```python
from build123d import *

# Parameters (mm, degrees)
SKETCH1_R           = 12.5
BOSS_EXTRUDE1_DEPTH = 8
SKETCH2_R           = 6.5
CUT_EXTRUDE1_DEPTH  = 4
SKETCH4_R           = 2
CUT_EXTRUDE3_DEPTH  = 4
SKETCH5_W           = 4
SKETCH5_H           = 6
CUT_EXTRUDE4_DEPTH  = 3
SKETCH3_R           = 1
CUT_EXTRUDE2_DEPTH  = 20.403607912
CHAMFER1_SIZE       = 1
CHAMFER2_SIZE       = 1


with BuildPart() as part:
    # Sketch1 → Boss-Extrude1 (new body)
    with BuildSketch(Plane(origin=(0, 0, 0), x_dir=(1, 0, 0), z_dir=(0, 1, 0))):
        with Locations(Location((0, 0, 0), (0, 0, 270))):
            Circle(SKETCH1_R)
    extrude(amount=BOSS_EXTRUDE1_DEPTH)

    # Sketch2 → Cut-Extrude1 (cut)
    with BuildSketch(Plane(origin=(0, 8, 0), x_dir=(1, 0, 0), z_dir=(0, 1, 0))):
        with Locations(Location((0, 0, 0), (0, 0, 270))):
            Circle(SKETCH2_R)
    extrude(amount=-CUT_EXTRUDE1_DEPTH, mode=Mode.SUBTRACT)

    # Sketch4 → Cut-Extrude3 (cut)
    with BuildSketch(Plane(origin=(0, 0, 0), x_dir=(-1, 0, 0), z_dir=(0, -1, 0))):
        with Locations(Location((0, 0, 0), (0, 0, 90))):
            Circle(SKETCH4_R)
    extrude(amount=-CUT_EXTRUDE3_DEPTH, mode=Mode.SUBTRACT)

    # Sketch5 → Cut-Extrude4 (cut)
    with BuildSketch(Plane(origin=(0, 0, 0), x_dir=(-1, 0, 0), z_dir=(0, -1, 0))):
        with Locations((0, -6.25)):
            Rectangle(SKETCH5_W, SKETCH5_H)
        Polygon((-10, -3.25), (-2, -3.25), (-2, 4e-09), (-2, 3.25), (-10, 3.25), align=None)
        with BuildLine():
            Line((-2, -3.25), (2, -3.25))
            Line((2, -3.25), (2, 0))
            ThreePointArc((2, 0), (-2e-09, -2), (-2, 4e-09))
            Line((-2, 4e-09), (-2, -3.25))
        make_face()
        with Locations((0, 6.25)):
            Rectangle(SKETCH5_W, SKETCH5_H)
        Polygon((2, -3.25), (10, -3.25), (10, 3.25), (2, 3.25), (2, 0), align=None)
        with BuildLine():
            ThreePointArc((-2, 4e-09), (2e-09, 2), (2, 0))
            Line((2, 0), (2, 3.25))
            Line((2, 3.25), (-2, 3.25))
            Line((-2, 3.25), (-2, 4e-09))
        make_face()
    extrude(amount=-CUT_EXTRUDE4_DEPTH, mode=Mode.SUBTRACT)

    # Sketch3 → Cut-Extrude2 (cut, through all)
    with BuildSketch(Plane(origin=(0, 8, 0), x_dir=(1, 0, 0), z_dir=(0, 1, 0))):
        with Locations(Location((7.778174593, 7.778174593, 0), (0, 0, 270))):
            Circle(SKETCH3_R)
        with Locations(Location((7.778174593, -7.778174593, 0), (0, 0, 270))):
            Circle(SKETCH3_R)
        with Locations(Location((-7.778174593, -7.778174593, 0), (0, 0, 270))):
            Circle(SKETCH3_R)
        with Locations(Location((-7.778174593, 7.778174593, 0), (0, 0, 270))):
            Circle(SKETCH3_R)
    extrude(amount=-CUT_EXTRUDE2_DEPTH, mode=Mode.SUBTRACT)

    # Chamfer1
    # the kernel refuses this chamfer: 1 mm, written as the material it takes off along each edge
    with BuildSketch(Plane(origin=(0, 0, 0), x_dir=(0, 0, 1), z_dir=(-1, 0, 0))) as chamfer1_piece_1:
        Polygon((12.5, CHAMFER1_SIZE), (12.5 - CHAMFER1_SIZE, 0), (12.5, 0), align=None)
    revolve(axis=Axis((0, 0, 0), (0, 1, 0)), mode=Mode.SUBTRACT)
    with BuildSketch(Plane(origin=(0, 8, 0), x_dir=(0, 0, 1), z_dir=(-1, 0, 0))) as chamfer1_piece_2:
        Polygon((12.5, -CHAMFER1_SIZE), (12.5 - CHAMFER1_SIZE, 0), (12.5, 0), align=None)
    revolve(axis=Axis((0, 8, 0), (0, 1, 0)), mode=Mode.SUBTRACT)
    with BuildSketch(Plane(origin=(0, 8, 0), x_dir=(0, 0, 1), z_dir=(-1, 0, 0))) as chamfer1_piece_3:
        Polygon((6.5 + CHAMFER1_SIZE, 0), (6.5, -CHAMFER1_SIZE), (6.5, 0), align=None)
    revolve(axis=Axis((0, 8, 0), (0, 1, 0)), mode=Mode.SUBTRACT)

    # Chamfer2
    chamfer2_edges = [part.edges().sort_by_distance(p)[0] for p in [
        (2, 1.5, -3.25),
        (-2, 1.5, -3.25),
        (-2, 1.5, 3.25),
        (2, 1.5, 3.25),
    ]]
    chamfer(chamfer2_edges, length=CHAMFER2_SIZE)


solid = part.part
```
Read the model definition and answer for the solid it produces. Units are mm, in the model's axes. A direction names the side the tool comes from. Give positions to 0.01 mm unless a question says otherwise; leave off trailing zeros. Write each loop counter-clockwise with the first axis right and the second up, starting at its lowest first coordinate (ties: lowest second). Pieces come first, ordered by that corner, then holes. Notation, with made-up numbers: (23, -16.5) - (57, -16.5) arc R18 ccw to (57, -3.5) - close; hole circle Ø7 at (34, 69.25). An arc over 180 degrees is marked (long way). Write item = value, one per line. Start each with the question number.
Item 1: A tool of negligible diameter and unlimited length cuts with its end or side. For faces 1 (the cylindrical face through (6.9, 4.1, -7.3)), 2 (the flat face through (0, 1, -9.25)), 3 (the cylindrical face through (-3.955, 5.521, -5.158)), from which of +Z, -Z, +X, -X, +Y, -Y can it reach the whole face along a straight path? Write none if from no direction.
Item 2: Find the intervals of material crossed by probe 1 along X at (y, z) = (4.95, 0); probe 2 along X at (y, z) = (1.75, -7.5); probe 3 along X at (y, z) = (0.75, -7.75), in increasing order. Write a range as [from, to].
Item 3: Find section B-B (z = 0). Give the vertices of the cut face in (x, y).
Item 4: Find section C-C (y = 2.25). Give the vertices of the cut face in (x, z), then the cut area to 3 significant figures.
Item 5: Find section A-A (x = 0). Give the vertices of the cut face in (y, z), then the cut area to 3 significant figures.
Item 6: The mould has two halves that part along X. Classify faces 4 (the flat face through (-8, 8, 0)), 5 (the conical face through (-10.344, 0.16, 5.38)), 6 (the flat face through (2, 1, -7)): +X half, -X half, draft (parallel to the pull), parting line (faces both ways), or undercut.
Item 7: Each of these flat-tipped pins is pushed along its axis until it touches: P1, Ø1.5, axis at y = 1.5, z = 5.5, coming from the +X side; P2, Ø10.5, axis at x = -3, z = 1, coming from the +Y side; P3, Ø6.5, axis at x = 0, z = 0, coming from the -Y side; P4, Ø4, axis at x = -5, y = 1.5, coming from the -Z side. Where does it stop, or does it pass through?
Response:
q1.face_1 = +Y, -Y
q1.face_2 = -Y
q1.face_3 = +Y
q2.probe_1 = [-12.5, -6.5], [6.5, 12.5]
q2.probe_2 = [-10, -8.74], [-6.82, -2], [2, 6.82], [8.74, 10]
q2.probe_3 = [-9.49, -8.78], [-6.78, -2], [2, 6.78], [8.78, 9.49]
q3.outline = (-12.5, 1) - (-11.5, 0) - (-10, 0) - (-10, 3) - (-2, 3) - (-2, 4) - (-6.5, 4) - (-6.5, 7) - (-7.5, 8) - (-11.5, 8) - (-12.5, 7) - close; (2, 3) - (10, 3) - (10, 0) - (11.5, 0) - (12.5, 1) - (12.5, 7) - (11.5, 8) - (7.5, 8) - (6.5, 7) - (6.5, 4) - (2, 4) - close
q4.outline = circle Ø25 at (0, 0); hole (-10, -3.25) - (-3, -3.25) - (-2, -4.25) - (-2, -9.25) - (2, -9.25) - (2, -4.25) - (3, -3.25) - (10, -3.25) - (10, 3.25) - (3, 3.25) - (2, 4.25) - (2, 9.25) - (-2, 9.25) - (-2, 4.25) - (-3, 3.25) - (-10, 3.25) - close; hole circle Ø2 at (-7.78, -7.78); hole circle Ø2 at (-7.78, 7.78); hole circle Ø2 at (7.78, -7.78); hole circle Ø2 at (7.78, 7.78)
q4.area = 298 mm²
q5.outline = (0, -11.5) - (1, -12.5) - (7, -12.5) - (8, -11.5) - (8, -7.5) - (7, -6.5) - (4, -6.5) - (4, -2) - (3, -2) - (3, -9.25) - (0, -9.25) - close; (0, 9.25) - (3, 9.25) - (3, 2) - (4, 2) - (4, 6.5) - (7, 6.5) - (8, 7.5) - (8, 11.5) - (7, 12.5) - (1, 12.5) - (0, 11.5) - close
q5.area = 85.5 mm²
q6.face_4 = draft
q6.face_5 = parting line
q6.face_6 = undercut
q7.P1 = 11.56
q7.P2 = 8
q7.P3 = 3
q7.P4 = -12.13
